For this review, use the dimensioned drawing (mm, ordinates from the lowest corner) and the shaded views. Round coordinates to 2 decimals unless told otherwise and drop trailing zeros. Loops run counter-clockwise (first coordinate to the right, second up) from the corner with the lowest first, then second, coordinate; pieces in that order, holes last. Notation, with made-up numbers: M 72,-38 L 87,-38 A23 cw 87,-18 Z; hole C 10.25,61 d1. An arc over 180 degrees is marked long. Answer as a JSON object with one key per item and string values. Group by question number.
Item 1: Consider section B-B (z = 59.5). Give the boundary of the cut face in (x, y), and give its area (3 significant figures).
Item 2: To check wall thickness, follow line 1 (Z direction, x = 172.5, y = 4); line 2 (X direction, y = 4.25, z = 132). State the ranges of each line that lie inside material, in increasing order.
Item 3: Consider section A-A (x = 59.5). Give the boundary of the cut face in (y, z).
Item 4: Insertion check: P1, Ø1.9, axis at x = 101.5, y = 4, coming from the -Z side; P2, Ø1.9, axis at x = 173, y = 2.5, coming from the +Z side; P3, Ø1.9, axis at y = 1.5, z = 31, coming from the -X side. Each pin has a flat end and moves straight along its axis. Give the tip position at first contact, or say it passes through.
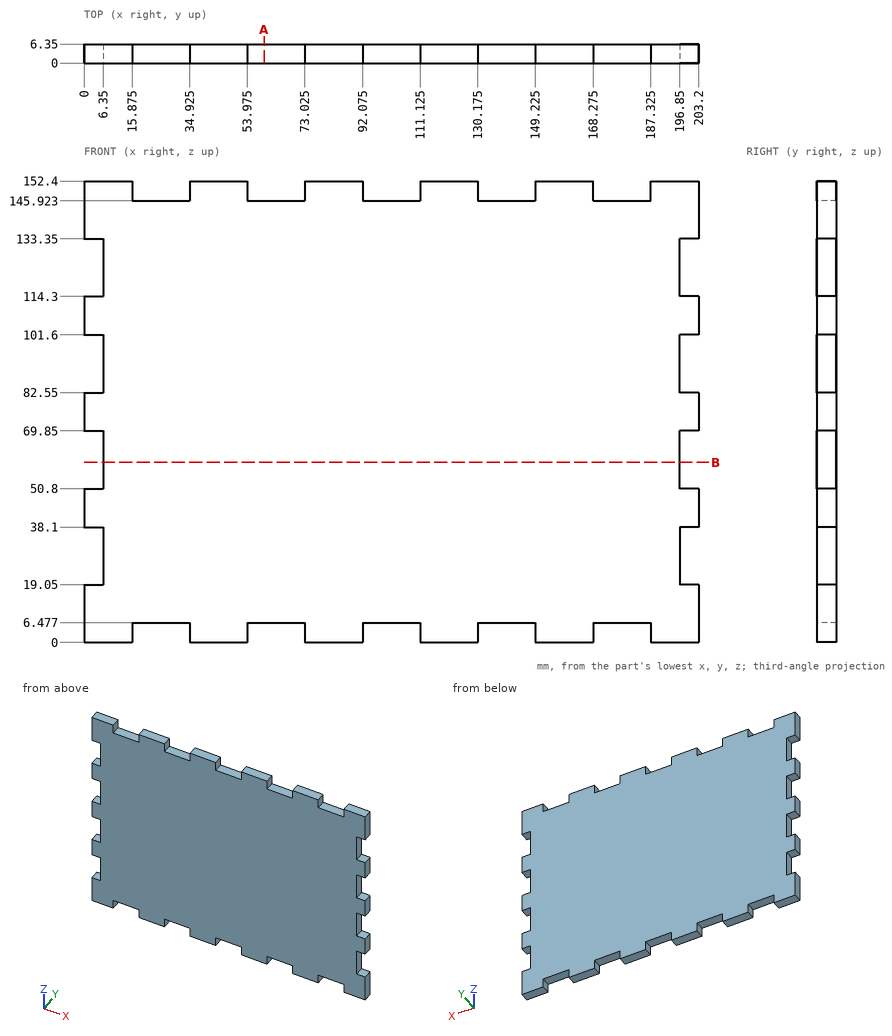
Geometry results:
{
 "1": {"outline": "M 6.35,0 L 196.85,0 L 196.85,6.35 L 6.35,6.35 Z", "area": "1,210 mm^2"},
 "2": {"line 1": "z = 6.48 to 145.92", "line 2": "x = 6.35 to 196.85"},
 "3": {"outline": "M 0,6.48 L 6.35,6.48 L 6.35,145.92 L 0,145.92 Z"},
 "4": {"P1": "stops at z = 6.48", "P2": "stops at z = 145.92", "P3": "stops at x = 6.35"}
}
